```python
from build123d import *
from OCP.BRepFilletAPI import BRepFilletAPI_MakeChamfer

# Parameters (mm, degrees)
ESQUISSE1_W             = 213
ESQUISSE1_H             = 80
BOSS_EXTRU_1_DEPTH      = 4
CHANFREIN1_SIZE         = 4
CHANFREIN1_SIZE_2       = 2.309401077
CONG_1_R                = 6.5
ESQUISSE2_R             = 1.5
ENL_V_MAT_EXTRU_1_DEPTH = 134.260084046
ENL_V_MAT_EXTRU_2_DEPTH = 134.260084046
CHANFREIN2_SIZE         = 1.5
ENL_V_MAT_EXTRU_3_DEPTH = 134.260084046
CONG_2_R                = 2


with BuildPart() as part:
    # Esquisse1 → Boss.-Extru.1 (new body)
    with BuildSketch(Plane.XY):
        with Locations((0, -40)):
            Rectangle(ESQUISSE1_W, ESQUISSE1_H)
    extrude(amount=BOSS_EXTRU_1_DEPTH)

    # Chanfrein1
    chanfrein1_edges_1 = [part.edges().sort_by_distance(p)[0] for p in [
        (-106.5, -40, 0),
    ]]
    chanfrein1_side_1 = [part.faces().sort_by_distance(p)[0] for p in [
        (-106.5, -40, 0.046188022),
    ]]
    chanfrein1_edges_2 = [part.edges().sort_by_distance(p)[0] for p in [
        (106.5, -40, 0),
    ]]
    chanfrein1_side_2 = [part.faces().sort_by_distance(p)[0] for p in [
        (106.5, -40, 0.046188022),
    ]]
    chanfrein1 = BRepFilletAPI_MakeChamfer(part.part.solid().wrapped)
    for e in chanfrein1_edges_1:
        chanfrein1.Add(CHANFREIN1_SIZE - 0.0001, CHANFREIN1_SIZE_2 - 0.0001, e.wrapped, chanfrein1_side_1[0].wrapped)
    for e in chanfrein1_edges_2:
        chanfrein1.Add(CHANFREIN1_SIZE - 0.0001, CHANFREIN1_SIZE_2 - 0.0001, e.wrapped, chanfrein1_side_2[0].wrapped)
    add(Compound.cast(chanfrein1.Shape()), mode=Mode.REPLACE)  # a hair under: the kernel refuses the full size

    # Congé1
    cong_1_edges = [part.edges().sort_by_distance(p)[0] for p in [
        (104.190698923, -40, 0),
        (-104.190698923, -40, 0),
    ]]
    fillet(cong_1_edges, radius=CONG_1_R)

    # Esquisse2 → Enlèv. mat.-Extru.1 (cut, through all)
    with BuildSketch(Plane(origin=(0, 0, 0), x_dir=(-1, 0, 0), z_dir=(0, 0, -1))):
        with Locations((-95, -40)):
            Circle(ESQUISSE2_R)
        with Locations(Location((95, -40, 0), (0, 0, 180))):
            Circle(ESQUISSE2_R)
        with Locations((0, -40)):
            Circle(ESQUISSE2_R)
    extrude(amount=-ENL_V_MAT_EXTRU_1_DEPTH, mode=Mode.SUBTRACT)

    # Esquisse3 → Enlèv. mat.-Extru.2 (cut, through all)
    with BuildSketch(Plane(origin=(0, 0, 0), x_dir=(1, 0, 0), z_dir=(0, 1, 0))):
        with BuildLine():
            Line((-89.5, -3.5), (-10.5, -3.5))
            ThreePointArc((-10.5, -3.5), (-10, -4), (-10.5, -4.5))
            Line((-10.5, -4.5), (-89.5, -4.5))
            ThreePointArc((-89.5, -4.5), (-90, -4), (-89.5, -3.5))
        make_face()
        with BuildLine():
            Line((10.5, -3.5), (89.5, -3.5))
            ThreePointArc((89.5, -3.5), (90, -4), (89.5, -4.5))
            Line((89.5, -4.5), (10.5, -4.5))
            ThreePointArc((10.5, -4.5), (10, -4), (10.5, -3.5))
        make_face()
    extrude(amount=-ENL_V_MAT_EXTRU_2_DEPTH, mode=Mode.SUBTRACT)

    # Chanfrein2
    chanfrein2_edges = [part.edges().sort_by_distance(p)[0] for p in [
        (96.5, -40, 0),
        (-96.5, -40, 0),
        (1.5, -40, 0),
    ]]
    chamfer(chanfrein2_edges, length=CHANFREIN2_SIZE)

    # Esquisse4 → Enlèv. mat.-Extru.3 (cut, through all)
    with BuildSketch(Plane(origin=(0, 0, 0), x_dir=(-1, 0, 0), z_dir=(0, 0, -1))):
        with BuildLine():
            Line((-87, -80), (-13, -80))
            ThreePointArc((-13, -80), (-17.630306208, -71.827984304), (-24.080128411, -65))
            Line((-24.080128411, -65), (-75.919871589, -65))
            ThreePointArc((-75.919871589, -65), (-82.369693792, -71.827984304), (-87, -80))
        make_face()
        with BuildLine():
            Line((87, -80), (13, -80))
            ThreePointArc((13, -80), (17.630306208, -71.827984304), (24.080128411, -65))
            Line((24.080128411, -65), (75.919871589, -65))
            ThreePointArc((75.919871589, -65), (82.369693792, -71.827984304), (87, -80))
        make_face()
    extrude(amount=-ENL_V_MAT_EXTRU_3_DEPTH, mode=Mode.SUBTRACT)

    # Congé2
    cong_2_edges = [part.edges().sort_by_distance(p)[0] for p in [
        (87, -80, 1.75),
        (75.919871589, -65, 1.75),
        (24.080128411, -65, 1.75),
        (13, -80, 1.75),
        (-75.919871589, -65, 1.75),
        (-87, -80, 1.75),
        (-13, -80, 1.75),
        (-24.080128411, -65, 1.75),
    ]]
    fillet(cong_2_edges, radius=CONG_2_R)


solid = part.part
```
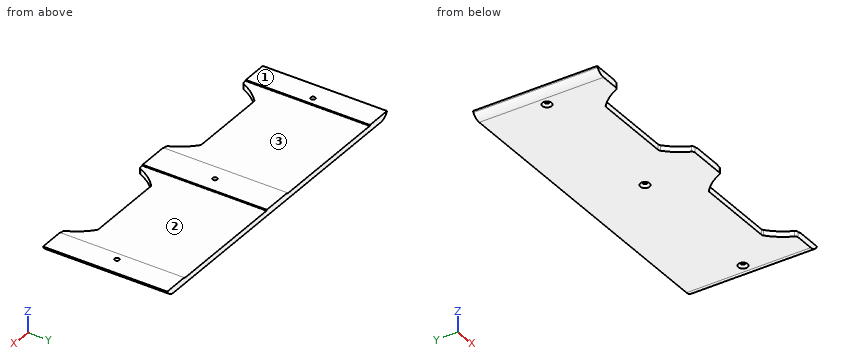
Verification items for the finished model (mm, model axes). Face numbers are marked on the shaded views. Round coordinates to 2 decimals unless told otherwise and drop trailing zeros. Order: outer loops, then holes, each group sorted by start corner. A loop starts at its lowest first (then second) coordinate and runs counter-clockwise, first axis right, second up. Notation, with made-up numbers: (-4.5, -37) -> (22.5, -37) arc R31 ccw to (22.5, -4) -> close; hole circle Ø5 at (62.5, 82). An arc over 180 degrees is marked (long way). Put each result on its own line as item: value. Start each with the question number.
(1) Section check D-D (x = 59). Enter the section's corners in (y, z).
(2) Section check A-A (y = -75). State how many separate pieces and enclosed holes the cut face has, then the cut area to 3 significant figures.
(3) Section check B-B (z = 2.15). Enter the section's corners in (x, y), then the cut area to 3 significant figures.
(4) Material ranges on line 1 along Y through (x, z) = (-95, 2.25); line 2 along X through (y, z) = (-73, 1.5); line 3 along Z through (x, y) = (-62, -32.5), recorded low to high.
(5) Depth check by flat-ended pin: pin 1 Ø1 at (x, z) = (-62.5, 1.5) entering from -Y; pin 2 Ø1.8 at (x, y) = (-95, -40) entering from +Z; pin 3 Ø5 at (x, y) = (49.5, -13.5) entering from +Z; pin 4 Ø2 at (y, z) = (-31, 1.5) entering from -X. Enter the tip coordinate at first touch or a pass-through.
(6) Draft check along X on the marked faces 1, 2 and 3. Enter one of: +X half, -X half, draft (parallel to the pull), parting line (faces both ways), or undercut.
Completed:
1. outline: (-65, 0) -> (0, 0) -> (0, 3.5) -> (-65, 3.5) -> close
2. separate pieces: 3
2. enclosed holes: 0
2. area: 276 mm2
3. outline: (-105.27, -80) -> (-88.31, -80) arc R2 ccw to (-86.49, -78.83) arc R39 cw to (-76.49, -65.49) arc R2 cw to (-75.19, -65) -> (-24.81, -65) arc R2 cw to (-23.51, -65.49) arc R39 cw to (-13.51, -78.83) arc R2 ccw to (-11.69, -80) -> (11.69, -80) arc R2 ccw to (13.51, -78.83) arc R39 cw to (23.51, -65.49) arc R2 cw to (24.81, -65) -> (75.19, -65) arc R2 cw to (76.49, -65.49) arc R39 cw to (86.49, -78.83) arc R2 ccw to (88.31, -80) -> (105.27, -80) -> (105.27, 0) -> (-105.27, 0) -> close; hole circle Ø3 at (-95, -40); hole circle Ø3 at (0, -40); hole circle Ø3 at (95, -40)
3. area: 14,900 mm2
4. line 1: y = -80 to -41.5, -38.5 to 0
4. line 2: x = -104.59 to -83.2, -16.8 to 16.8, 83.2 to 104.59
4. line 3: z = 0 to 3.5
5. pin 1: stops at y = -65
5. pin 2: passes through
5. pin 3: stops at z = 3.5
5. pin 4: stops at x = -105.56
6. face 1: draft
6. face 2: undercut
6. face 3: undercut
